Here's how the part is built. I have some questions about the finished solid (model axes, mm). Round coordinates to 2 decimals unless told otherwise and drop trailing zeros. Order: outer loops, then holes, each group sorted by start corner. A loop starts at its lowest first (then second) coordinate and runs counter-clockwise, first axis right, second up. Notation, with made-up numbers: (32, 25) -> (59, 25) arc R29 cw to (59, 52) -> close; hole circle Ø7 at (2.25, -4). An arc over 180 degrees is marked (long way). Use a Markdown table: item, result. Add a question column.
(1) I'm going to push flat-ended pins straight in: P1, Ø10, axis at y = 43.5, z = 3, coming from the -X side; P2, Ø6, axis at x = 5.5, z = 16, coming from the +Y side; P3, Ø5, axis at x = 18.5, z = 22, coming from the -Y side. Where does each tip first touch, or does it pass through?
(2) I want a section at A-A, the plane y = 39. Please give me the cut outline in (x, z).
(3) I want a section at C-C, the plane x = 4.5. Please give me the cut outline in (y, z), then the cut area to 3 significant figures.
(4) If I drill on probe 1 along X at (y, z) = (16.5, 18); probe 2 along Y at (x, z) = (-23, 4.75); probe 3 along X at (y, z) = (-3, 19.25), over which ranges is the centre line in solid material (lowest first)?
from build123d import *

# Parameters (mm, degrees)
F1_DEPTH = 25.4


with BuildPart() as f1:
    # F0 (on Top) → F1 (new body)
    with BuildSketch(Plane.XY):
        with BuildLine():
            ThreePointArc((-13.8794476694, 23.9851492257), (0.0388587333, 27.7114586585), (13.946659894, 23.9461297245))
            ThreePointArc((13.946659894, 23.9461297245), (13.9466804124, 23.9656394703), (13.9466872518, 23.9851492257))
            ThreePointArc((13.9466872518, 23.9851492257), (-13.9264962423, 51.8112443718), (-41.7054234906, 23.8910522142))
            ThreePointArc((-41.7054234906, 23.8910522142), (-27.805115023, 27.6876127299), (-13.8794476694, 23.9851492257))
        make_face()
        with BuildLine():
            ThreePointArc((-27.7110248308, -0.1598555968), (-24.0455227676, 13.7745884083), (-13.8794476694, 23.9851492257))
            ThreePointArc((-13.8794476694, 23.9851492257), (-27.805115023, 27.6876127299), (-41.7054234906, 23.8910522142))
            ThreePointArc((-41.7054234906, 23.8910522142), (-37.9304241934, 9.9907105841), (-27.7110248308, -0.1598555968))
        make_face()
        with BuildLine():
            ThreePointArc((-0.0241009827, -0.1462235666), (10.192242734, 10.026370419), (13.946659894, 23.9461297245))
            ThreePointArc((13.946659894, 23.9461297245), (0.0388587333, 27.7114586585), (-13.8794476694, 23.9851492257))
            ThreePointArc((-13.8794476694, 23.9851492257), (-3.7365930705, 13.8498078951), (-0.0237148649, 0))
            ThreePointArc((-0.0237148649, 0), (-0.0238113945, -0.0731120382), (-0.0241009827, -0.1462235666))
        make_face()
        with BuildLine():
            ThreePointArc((-0.0237148649, 0), (-3.7365930705, 13.8498078951), (-13.8794476694, 23.9851492257))
            ThreePointArc((-13.8794476694, 23.9851492257), (-24.0455227676, 13.7745884083), (-27.7110248308, -0.1598555968))
            ThreePointArc((-27.7110248308, -0.1598555968), (-13.8657470984, -3.8409823227), (-0.0241009827, -0.1462235666))
            ThreePointArc((-0.0241009827, -0.1462235666), (-0.0238113945, -0.0731120382), (-0.0237148649, 0))
        make_face()
        with BuildLine():
            ThreePointArc((-27.7110248308, -0.1598555968), (-23.9656630374, -13.9130674606), (-13.8794476694, -23.9851492257))
            ThreePointArc((-13.8794476694, -23.9851492257), (-3.7732483133, -13.9130674606), (-0.0241009827, -0.1462235666))
            ThreePointArc((-0.0241009827, -0.1462235666), (-13.8657470984, -3.8409823227), (-27.7110248308, -0.1598555968))
        make_face()
        with BuildLine():
            ThreePointArc((-13.8794476694, -23.9851492257), (13.8438855193, -24.0056927563), (27.7114859036, 0))
            ThreePointArc((27.7114859036, 0), (24.0250818941, 13.810209664), (13.946659894, 23.9461297245))
            ThreePointArc((13.946659894, 23.9461297245), (10.192242734, 10.026370419), (-0.0241009827, -0.1462235666))
            ThreePointArc((-0.0241009827, -0.1462235666), (-3.7732483133, -13.9130674606), (-13.8794476694, -23.9851492257))
        make_face()
        with BuildLine():
            ThreePointArc((-41.7054234906, 23.8910522142), (-51.6497234938, -13.9130674606), (-13.8794476694, -23.9851492257))
            ThreePointArc((-13.8794476694, -23.9851492257), (-23.9656630374, -13.9130674606), (-27.7110248308, -0.1598555968))
            ThreePointArc((-27.7110248308, -0.1598555968), (-37.9304241934, 9.9907105841), (-41.7054234906, 23.8910522142))
        make_face()
    extrude(amount=F1_DEPTH)


solid = f1.part
Taken from the geometry:
| question | item | result |
|---|---|---|
| 1 | P1 | stops at x = -37.62 |
| 1 | P2 | stops at y = 46.48 |
| 1 | P3 | stops at y = -22.63 |
| 2 | outline | (-37.31, 0) -> (9.55, 0) -> (9.55, 25.4) -> (-37.31, 25.4) -> close |
| 3 | outline | (-27.34, 0) -> (44.88, 0) -> (44.88, 25.4) -> (-27.34, 25.4) -> close |
| 3 | area | 1,830 mm2 |
| 4 | probe 1 | x = -49.95 to 22.26 |
| 4 | probe 2 | y = -27.28 to 50.27 |
| 4 | probe 3 | x = -55.24 to 27.55 |
